The listing builds one solid part. Answer for the finished solid, in the listing's coordinates (mm). Face numbers are marked on the shaded views. A direction names the side the tool comes from. Round coordinates to 2 decimals unless told otherwise and drop trailing zeros. Loops run counter-clockwise (first coordinate to the right, second up) from the corner with the lowest first, then second, coordinate; pieces in that order, holes last. Notation, with made-up numbers: (48.5, 71.5) -> (94.5, 71.5) arc R5 cw to (94.5, 76.5) -> close; hole circle Ø2 at (57, -26). An arc over 180 degrees is marked (long way). One line per question, with ' | ' between items.
from build123d import *

# Parameters (mm, degrees)
F1_DEPTH = 35
F2_R     = 1.6
F3_DEPTH = 28.5
F5_DEPTH = 2


with BuildPart() as f1:
    # F0 (on Right) → F1 (new body)
    with BuildSketch(Plane.YZ):
        with BuildLine():
            Line((0, 0), (0, 28.5))
            Line((0, 28.5), (-60.2, 28.5))
            Line((-60.2, 28.5), (-60.2, 0))
            Line((-60.2, 0), (-55.2, 0))
            Line((-55.2, 0), (-55.2, 10))
            Line((-55.2, 10), (-45.2, 10))
            ThreePointArc((-45.2, 10), (-31.35, 24), (-17.5, 10))
            Line((-17.5, 10), (-5, 10))
            Line((-5, 10), (-5, 0))
            Line((-5, 0), (0, 0))
        make_face()
    extrude(amount=F1_DEPTH)

    # F2 (on face) → F3 (cut, through all)
    with BuildSketch(Plane.XY.offset(28.5)):
        with Locations((4.5, -3)):
            Circle(F2_R)
        with Locations((30.5, -3)):
            Circle(F2_R)
        with Locations((17.5, -57.2)):
            Circle(F2_R)
    extrude(amount=-F3_DEPTH, mode=Mode.SUBTRACT)

    # F4 (on face) → F5 (cut)
    with BuildSketch(Plane.XY.offset(28.5)):
        Polygon((2.796817, -5.95), (6.203183, -5.95), (7.906367, -3), (6.203183, -0.05), (2.796817, -0.05), (1.093633, -3), align=None)
        Polygon((28.796817, -5.95), (32.203183, -5.95), (33.906367, -3), (32.203183, -0.05), (28.796817, -0.05), (27.093633, -3), align=None)
        Polygon((19.203183, -54.25), (15.796817, -54.25), (14.093633, -57.2), (15.796817, -60.15), (19.203183, -60.15), (20.906367, -57.2), align=None)
    extrude(amount=-F5_DEPTH, mode=Mode.SUBTRACT)


solid = f1.part
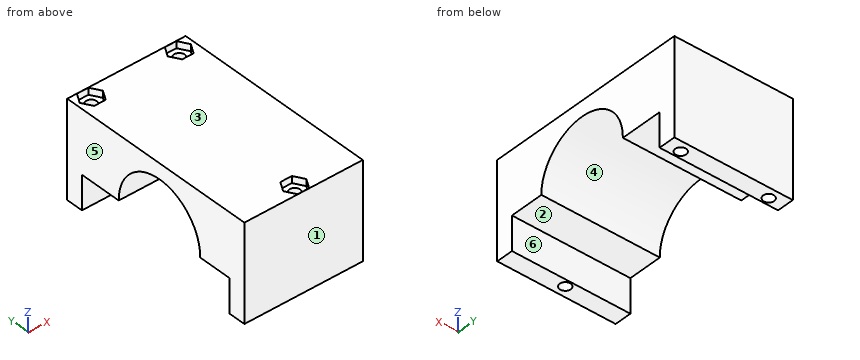
Q1. For a pull along Y with two mould halves and no side action, classify the marked faces 1, 2, 3 and 4 as pulls with the +Y half, pulls with the -Y half, needs draft (parallel to the pull), parting line crosses it, or undercut.
Numbers:
face 1: pulls with the -Y half | face 2: undercut | face 3: needs draft | face 4: undercut
Q2. A cutting plane is placed at C-C on x = 10. Give the vertices of the cut face in (y, z), plus the area to 3 significant figures.
Numbers:
outline: (-60.2, 0) -> (-55.2, 0) -> (-55.2, 10) -> (-45.2, 10) arc R13.85 cw (long way) to (-17.5, 10) -> (-5, 10) -> (-5, 0) -> (0, 0) -> (0, 28.5) -> (-60.2, 28.5) -> close | area: 908 mm^2
Q3. A cutting plane is placed at A-A on z = 15.25. Give the vertices of the cut face in (x, y), plus the area to 3 significant figures.
Numbers:
outline: (0, -60.2) -> (35, -60.2) -> (35, -44.23) -> (0, -44.23) -> close; (0, -18.47) -> (35, -18.47) -> (35, 0) -> (0, 0) -> close; hole circle Ø3.2 at (4.5, -3); hole circle Ø3.2 at (17.5, -57.2); hole circle Ø3.2 at (30.5, -3) | area: 1,180 mm^2
Q4. For the marked faces 5 and 6, determine the directions among +Z, -Z, +X, -X, +Y, -Y from which every point of the face is accessible in a straight line to the end or side of a thin tool.
Numbers:
face 5: +Z, -Z, -X, +Y, -Y | face 6: -Z, +X, -X
Q5. A cutting plane is placed at D-D on z = 20. Give the vertices of the cut face in (x, y).
Numbers:
outline: (0, -60.2) -> (35, -60.2) -> (35, -41.09) -> (0, -41.09) -> close; (0, -21.61) -> (35, -21.61) -> (35, 0) -> (0, 0) -> close; hole circle Ø3.2 at (4.5, -3); hole circle Ø3.2 at (17.5, -57.2); hole circle Ø3.2 at (30.5, -3)
Q6. Given pin 1 Ø4 at (x, y) = (25.5, -25) entering from -Z; pin 2 Ø4.5 at (x, y) = (18, -57) entering from +Z; pin 3 Ø3 at (x, y) = (4.5, -3) entering from -Z, each flat-ended and moving along its own axis, determine where each tip first touches the part or whether it passes through.
Numbers:
pin 1: z = 21.2 | pin 2: z = 26.5 | pin 3: through
Q7. A cutting plane is placed at B-B on x = 17.5. Give the vertices of the cut face in (y, z).
Numbers:
outline: (-60.2, 0) -> (-58.8, 0) -> (-58.8, 26.5) -> (-60.15, 26.5) -> (-60.15, 28.5) -> (-60.2, 28.5) -> close; (-55.6, 0) -> (-55.2, 0) -> (-55.2, 10) -> (-45.2, 10) arc R13.85 cw (long way) to (-17.5, 10) -> (-5, 10) -> (-5, 0) -> (0, 0) -> (0, 28.5) -> (-54.25, 28.5) -> (-54.25, 26.5) -> (-55.6, 26.5) -> close
Q8. Find the intervals of material crossed by line 1 (Y direction, x = 5, z = 1.75); line 2 (Y direction, x = 18.5, z = 12); line 3 (Z direction, x = 27.5, y = -44), in increasing order. Write a range as from..to.
Numbers:
line 1: -60.2..-55.2, -5..-4.52, -1.48..0 | line 2: -60.2..-58.45, -55.95..-45.08, -17.62..0 | line 3: 15.79..28.5
